```python
from build123d import *

# Parameters (mm, degrees)
SKETCH1_W                                       = 56
SKETCH1_H                                       = 104
BOSS_EXTRUDE1_DEPTH                             = 29.6
SKETCH2_W                                       = 56
SKETCH2_H                                       = 104
BOSS_EXTRUDE2_DEPTH                             = 5
FILLET1_R                                       = 2
SKETCH3_W                                       = 25
SKETCH3_H                                       = 21.6
CUT_EXTRUDE1_DEPTH                              = 53
CUT_EXTRUDE1_DEPTH_BACK                         = 53
FILLET2_R                                       = 2
FILLET3_R                                       = 6.5
CSK_FOR_M5_FLAT_HEAD_MACHINE_SCREW1_D           = 5.8
CSK_FOR_M5_FLAT_HEAD_MACHINE_SCREW1_CSINK_D     = 10.4
CSK_FOR_M5_FLAT_HEAD_MACHINE_SCREW1_CSINK_ANGLE = 90
CHAMFER1_SIZE                                   = 0.8


with BuildPart() as part:
    # Sketch1 → Boss-Extrude1 (new body)
    with BuildSketch(Plane.XY):
        Rectangle(SKETCH1_W, SKETCH1_H)
        with BuildLine():
            Line((25, 24), (25, -24))
            ThreePointArc((25, -24), (0, -49), (-25, -24))
            Line((-25, -24), (-25, 24))
            ThreePointArc((-25, 24), (0, 49), (25, 24))
        make_face(mode=Mode.SUBTRACT)
    extrude(amount=BOSS_EXTRUDE1_DEPTH)

    # Sketch2 → Boss-Extrude2 (add)
    with BuildSketch(Plane(origin=(0, 0, 0), x_dir=(-1, 0, 0), z_dir=(0, 0, -1))):
        Rectangle(SKETCH2_W, SKETCH2_H)
        with BuildLine():
            Line((-15, 24), (-15, -24))
            ThreePointArc((-15, -24), (0, -39), (15, -24))
            Line((15, -24), (15, 24))
            ThreePointArc((15, 24), (0, 39), (-15, 24))
        make_face(mode=Mode.SUBTRACT)
    extrude(amount=BOSS_EXTRUDE2_DEPTH)

    # Fillet1
    fillet1_edges = [part.edges().sort_by_distance(p)[0] for p in [
        (0, 49, 0),
        (-25, 0, 0),
        (0, -49, 0),
        (25, 0, 0),
        (0, 39, 0),
        (15, 0, 0),
        (0, -39, 0),
        (-15, 0, 0),
    ]]
    fillet(fillet1_edges, radius=FILLET1_R)

    # Sketch3 → Cut-Extrude1 (cut, two sides)
    with BuildSketch(Plane(origin=(0, 0, 0), x_dir=(1, 0, 0), z_dir=(0, 1, 0))) as cut_extrude1_sk:
        with Locations((0, -18.8)):
            Rectangle(SKETCH3_W, SKETCH3_H)
    extrude(amount=CUT_EXTRUDE1_DEPTH, mode=Mode.SUBTRACT)
    extrude(cut_extrude1_sk.sketch, amount=-CUT_EXTRUDE1_DEPTH_BACK, mode=Mode.SUBTRACT)

    # Fillet2
    fillet2_edges = [part.edges().sort_by_distance(p)[0] for p in [
        (-12.5, 48.825317547, 29.6),
        (-12.5, 48.825317547, 8),
        (12.5, 48.825317547, 8),
        (12.5, 48.825317547, 29.6),
        (-12.5, -48.825317547, 29.6),
        (-12.5, -48.825317547, 8),
        (12.5, -48.825317547, 8),
        (12.5, -48.825317547, 29.6),
    ]]
    fillet(fillet2_edges, radius=FILLET2_R)

    # Fillet3
    fillet3_edges = [part.edges().sort_by_distance(p)[0] for p in [
        (28, -52, 12.3),
        (-28, -52, 12.3),
        (-28, 52, 12.3),
        (28, 52, 12.3),
    ]]
    fillet(fillet3_edges, radius=FILLET3_R)

    # CSK for M5 Flat Head Machine Screw1 (through all)
    with Locations(Plane(origin=(21.5, 45.5, -5), x_dir=(-1, 0, 0), z_dir=(0, 0, -1))):
        with Locations((0, 0), (43, -91)):
            CounterSinkHole(CSK_FOR_M5_FLAT_HEAD_MACHINE_SCREW1_D / 2, CSK_FOR_M5_FLAT_HEAD_MACHINE_SCREW1_CSINK_D / 2, counter_sink_angle=CSK_FOR_M5_FLAT_HEAD_MACHINE_SCREW1_CSINK_ANGLE)

    # Chamfer1
    chamfer1_edges = [part.edges().sort_by_distance(p)[0] for p in [
        (-28, 0, -5),
        (0, 52, -5),
        (28, 0, -5),
        (0, -52, -5),
        (26.096194078, -50.096194078, -5),
        (26.096194078, 50.096194078, -5),
        (-26.096194078, -50.096194078, -5),
        (-26.096194078, 50.096194078, -5),
        (0, 39, -5),
        (15, 0, -5),
        (0, -39, -5),
        (-15, 0, -5),
    ]]
    chamfer(chamfer1_edges, length=CHAMFER1_SIZE)


solid = part.part
```
CAD build for the part. Positions are in the model's coordinates, mm. A direction names the side the tool comes from. Round coordinates to 2 decimals unless told otherwise and drop trailing zeros. Write each loop counter-clockwise with the first axis right and the second up, starting at its lowest first coordinate (ties: lowest second). Pieces come first, ordered by that corner, then holes. Notation, with made-up numbers: (36, 8) - (81, 8) arc R8 cw to (81, 17) - close; hole circle Ø3 at (-17.5, -0.75). An arc over 180 degrees is marked (long way). Return JSON: item names as keys, results as strings. Group by question number.
Item 1: Probe probe 1 along X at (y, z) = (-23, 28); probe 2 along X at (y, z) = (45, 22); probe 3 along X at (y, z) = (-3.5, -3). List the from-to ranges inside material, lowest first.
Item 2: Flat gauge pins, fed straight in: pin 1 Ø1.9 at (y, z) = (48, 20) entering from -X; pin 2 Ø5 at (y, z) = (-48.5, 22) entering from +X; pin 3 Ø6 at (x, y) = (0.5, -50) entering from +Z. Where does each tip first touch, or does it go through?
Item 3: 3-axis set-ups, long thin cutter, end or side, ignore diameter. For faces 5 (the face through (-25.583, -49.674, -4.861)), 6 (the face through (15.6, -0.34, -0.57)), 7 (the face through (0, 39, -3)), 8 (the face through (26, 1, 29.6)), 9 (the face through (-11.93, -48.87, 8.6)): which of +Z, -Z, +X, -X, +Y, -Y reach the whole face in a straight line?
Item 4: Mould opens along Y. For faces 1 (the face through (-25.674, 49.583, -4.861)), 2 (the face through (-25, 0, 16)), 3 (the face through (-26, 12, 29.6)), 4 (the face through (-26.045, -50.146, 12.463)) say: +Y half, -Y half, draft (parallel to the pull), parting line (faces both ways), or undercut.
Item 5: Band-saw the part on B-B on x = 0. List the corners of the cut face in (y, z).
Item 6: Band-saw the part on D-D on z = 5. List the corners of the cut face in (x, y).
Item 7: Band-saw the part on A-A on z = 17.5. List the corners of the cut face in (x, y).
Item 8: Band-saw the part on C-C on y = 14. List the corners of the cut face in (x, z), plus the area to 3 significant figures.
Resolved:
{
 "1": {"probe 1": "x = -28 to -25, 25 to 28", "probe 2": "x = -28 to -13.56, 13.56 to 18.64, 24.36 to 28", "probe 3": "x = -28 to -15, 15 to 28"},
 "2": {"pin 1": "stops at x = -27.81", "pin 2": "stops at x = 27.98", "pin 3": "stops at z = 8"},
 "3": {"face 5": "-Z, -X, -Y", "face 6": "+Z", "face 7": "+Z, -Z", "face 8": "+Z, +X, -X, +Y, -Y", "face 9": "+Z, +Y, -Y"},
 "4": {"face 1": "+Y half", "face 2": "undercut", "face 3": "draft", "face 4": "-Y half"},
 "5": {"outline": "(-52, -4.2) - (-51.2, -5) - (-39.8, -5) - (-39, -4.2) - (-39, -2) arc R2 ccw to (-41, 0) - (-47, 0) arc R2 cw to (-49, 2) - (-49, 8) - (-52, 8) - close; (39, -4.2) - (39.8, -5) - (51.2, -5) - (52, -4.2) - (52, 8) - (49, 8) - (49, 2) arc R2 cw to (47, 0) - (41, 0) arc R2 ccw to (39, -2) - close"},
 "6": {"outline": "(-28, -45.5) arc R6.5 ccw to (-21.5, -52) - (21.5, -52) arc R6.5 ccw to (28, -45.5) - (28, 45.5) arc R6.5 ccw to (21.5, 52) - (-21.5, 52) arc R6.5 ccw to (-28, 45.5) - close; hole (-25, -24) arc R25 ccw to (25, -24) - (25, 24) arc R25 ccw to (-25, 24) - close; hole circle Ø5.8 at (-21.5, -45.5); hole circle Ø5.8 at (21.5, 45.5)"},
 "7": {"outline": "(-28, -45.5) arc R6.5 ccw to (-21.5, -52) - (-12.5, -52) - (-12.5, -45.65) arc R25 cw to (-25, -24) - (-25, 24) arc R25 cw to (-12.5, 45.65) - (-12.5, 52) - (-21.5, 52) arc R6.5 ccw to (-28, 45.5) - close; (12.5, -52) - (21.5, -52) arc R6.5 ccw to (28, -45.5) - (28, 45.5) arc R6.5 ccw to (21.5, 52) - (12.5, 52) - (12.5, 45.65) arc R25 cw to (25, 24) - (25, -24) arc R25 cw to (12.5, -45.65) - close; hole circle Ø5.8 at (-21.5, -45.5); hole circle Ø5.8 at (21.5, 45.5)"},
 "8": {"outline": "(-28, -4.2) - (-27.2, -5) - (-15.8, -5) - (-15, -4.2) - (-15, -2) arc R2 ccw to (-17, 0) - (-23, 0) arc R2 cw to (-25, 2) - (-25, 29.6) - (-28, 29.6) - close; (15, -4.2) - (15.8, -5) - (27.2, -5) - (28, -4.2) - (28, 29.6) - (25, 29.6) - (25, 2) arc R2 cw to (23, 0) - (17, 0) arc R2 ccw to (15, -2) - close", "area": "306 mm²"}
}
